from build123d import *

# Parameters (mm, degrees)
CHAMFER_1_SIZE      = 0.5
FILLET_1_R          = 1
CUT_EXTRUDE_1_REACH = 24.233
SKETCH_3_R          = 4.5
SKETCH_3_R_2        = 4.3
CUT_EXTRUDE_2_DEPTH = 0.2


with BuildPart() as part:
    # 草图1 → 旋转1 (revolve)
    with BuildSketch(Plane(origin=(0, 0, 0), x_dir=(0, 0, -1), z_dir=(1, 0, 0)), mode=Mode.PRIVATE) as revolve_1_sk:
        Polygon((-3.65, 0), (-4.5, 0), (-4.5, 16.4), (-6.25, 16.4), (-6.25, 20.4), (-1.7, 20.4), (-1.7, 15.4), (-3.65, 15.4), align=None)
    revolve(revolve_1_sk.sketch.rotate(Axis((0, 0, 0), (0, 1, 0)), 180), axis=Axis((0, 0, 0), (0, 1, 0)))

    # 倒角1
    chamfer_1_edges = [part.edges().sort_by_distance(p)[0] for p in [
        (0, 0, 3.65),
    ]]
    chamfer(chamfer_1_edges, length=CHAMFER_1_SIZE)

    # 圆角1
    fillet_1_edges = [part.edges().sort_by_distance(p)[0] for p in [
        (0, 16.4, 4.5),
    ]]
    fillet(fillet_1_edges, radius=FILLET_1_R)

    # 草图2 → 切除-拉伸1 (cut, up to next)
    with BuildSketch(Plane(origin=(0, 20.4, 0), x_dir=(1, 0, 0), z_dir=(0, 1, 0)), mode=Mode.PRIVATE) as cut_extrude_1_sk1:
        with BuildLine():
            Line((-5.75, 2.449489743), (-5.75, -2.449489743))
            ThreePointArc((-5.75, -2.449489743), (-6.25, 0), (-5.75, 2.449489743))
        make_face()
    cut_extrude_1_tool1 = extrude(cut_extrude_1_sk1.sketch, amount=-CUT_EXTRUDE_1_REACH, mode=Mode.PRIVATE) & part.part
    # 草图2 → 切除-拉伸1 (cut, up to next)
    with BuildSketch(Plane(origin=(0, 20.4, 0), x_dir=(1, 0, 0), z_dir=(0, 1, 0)), mode=Mode.PRIVATE) as cut_extrude_1_sk2:
        with BuildLine():
            Line((5.75, 2.449489743), (5.75, -2.449489743))
            ThreePointArc((5.75, -2.449489743), (6.25, 0), (5.75, 2.449489743))
        make_face()
    cut_extrude_1_tool2 = extrude(cut_extrude_1_sk2.sketch, amount=-CUT_EXTRUDE_1_REACH, mode=Mode.PRIVATE) & part.part
    add(cut_extrude_1_tool1.solids().sort_by_distance((-5.950702, 20.4, 0))[0], mode=Mode.SUBTRACT)
    add(cut_extrude_1_tool2.solids().sort_by_distance((5.950702, 20.4, 0))[0], mode=Mode.SUBTRACT)

    # 草图3 → 切除-拉伸2 (cut)
    with BuildSketch(Plane(origin=(0, 20.4, 0), x_dir=(1, 0, 0), z_dir=(0, 1, 0))):
        with Locations(Location((0, 0, 0), (0, 0, 90))):
            Circle(SKETCH_3_R)
        with Locations(Location((0, 0, 0), (0, 0, 270))):
            Circle(SKETCH_3_R_2, mode=Mode.SUBTRACT)
    extrude(amount=-CUT_EXTRUDE_2_DEPTH, mode=Mode.SUBTRACT)


solid = part.part
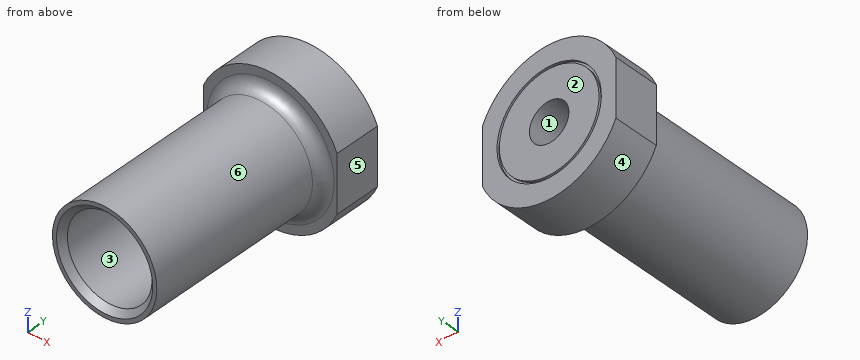
CAD build for the part. Positions are in the model's coordinates, mm. Face numbers are marked on the shaded views. A direction names the side the tool comes from. Give positions to 0.01 mm unless a question says otherwise; leave off trailing zeros. Order: outer loops, then holes, each group sorted by start corner. A loop starts at its lowest first (then second) coordinate and runs counter-clockwise, first axis right, second up. Notation, with made-up numbers: (-27, 12) - (2, 12) arc R14 ccw to (2, 37) - close; hole circle Ø10 at (-20.75, 9.5). An arc over 180 degrees is marked (long way). Answer in a Markdown table with one row per item.
1. Probe probe 1 along X at (y, z) = (11.75, 0); probe 2 along X at (y, z) = (16.8, 0); probe 3 along Y at (x, z) = (3, 2). List the from-to ranges inside material, lowest first. Write a range as [from, to].
Data:
| item | result |
|---|---|
| probe 1 | x = [-4.5, -3.65], [3.65, 4.5] |
| probe 2 | x = [-5.75, -1.7], [1.7, 5.75] |
| probe 3 | y = [15.4, 20.4] |
2. Saw through at A-A, the plane x = 0. Give the cut face in (y, z), plus the area to 3 significant figures.
Data:
| item | result |
|---|---|
| outline | (0, -4.5) - (15.4, -4.5) arc R1 cw to (16.4, -5.5) - (16.4, -6.25) - (20.4, -6.25) - (20.4, -4.5) - (20.2, -4.5) - (20.2, -4.3) - (20.4, -4.3) - (20.4, -1.7) - (15.4, -1.7) - (15.4, -3.65) - (0.5, -3.65) - (0, -4.15) - close; (0, 4.15) - (0.5, 3.65) - (15.4, 3.65) - (15.4, 1.7) - (20.4, 1.7) - (20.4, 4.3) - (20.2, 4.3) - (20.2, 4.5) - (20.4, 4.5) - (20.4, 6.25) - (16.4, 6.25) - (16.4, 5.5) arc R1 cw to (15.4, 4.5) - (0, 4.5) - close |
| area | 68.3 mm² |
3. Saw through at D-D, the plane z = 5.75. Give the cut face in (x, y).
Data:
| item | result |
|---|---|
| outline | (-2.45, 16.4) - (2.45, 16.4) - (2.45, 20.4) - (-2.45, 20.4) - close |
4. Tool access for the marked faces 5 and 6: list every direction of +Z, -Z, +X, -X, +Y, -Y with a clear straight run to the whole face (end or side of a thin tool).
Data:
| item | result |
|---|---|
| face 5 | +Z, -Z, +X, +Y, -Y |
| face 6 | -Y |
5. Pull direction Z, two halves, no side cores. Call the marked faces 1, 2, 3 and 4: pulls with the +Z half, pulls with the -Z half, needs draft (parallel to the pull), parting line crosses it, or undercut.
Data:
| item | result |
|---|---|
| face 1 | undercut |
| face 2 | needs draft |
| face 3 | undercut |
| face 4 | pulls with the -Z half |
6. Saw through at B-B, the plane z = 0. Give the cut face in (x, y), plus the area to 3 significant figures.
Data:
| item | result |
|---|---|
| outline | (-5.75, 16.4) - (-5.5, 16.4) arc R1 cw to (-4.5, 15.4) - (-4.5, 0) - (-4.15, 0) - (-3.65, 0.5) - (-3.65, 15.4) - (-1.7, 15.4) - (-1.7, 20.4) - (-4.3, 20.4) - (-4.3, 20.2) - (-4.5, 20.2) - (-4.5, 20.4) - (-5.75, 20.4) - close; (1.7, 15.4) - (3.65, 15.4) - (3.65, 0.5) - (4.15, 0) - (4.5, 0) - (4.5, 15.4) arc R1 cw to (5.5, 16.4) - (5.75, 16.4) - (5.75, 20.4) - (4.5, 20.4) - (4.5, 20.2) - (4.3, 20.2) - (4.3, 20.4) - (1.7, 20.4) - close |
| area | 64.3 mm² |
7. Saw through at C-C, the plane y = 19.25. Give the cut face in (x, z), plus the area to 3 significant figures.
Data:
| item | result |
|---|---|
| outline | (-5.75, -2.45) arc R6.25 ccw to (5.75, -2.45) - (5.75, 2.45) arc R6.25 ccw to (-5.75, 2.45) - close; hole circle Ø3.4 at (0, 0) |
| area | 110 mm² |
8. Flat gauge pins, fed straight in: pin 1 (3 mm diameter, centred on x = 1, y = 7, fed in from -Z); pin 2 (1 mm diameter, centred on x = 2.5, y = 5.5, fed in from +Z); pin 3 (2.5 mm diameter, centred on x = -0.5, z = 0.5, fed in from +Y); pin 4 (2 mm diameter, centred on x = -2.5, z = 0, fed in from -Y). Where does each tip first touch, or does it go through?
Data:
| item | result |
|---|---|
| pin 1 | stops at z = -4.5 |
| pin 2 | stops at z = 4.03 |
| pin 3 | stops at y = 20.4 |
| pin 4 | stops at y = 15.4 |
